```python
from build123d import *

# Parameters (mm, degrees)
F0_R            = 40
F2_DEPTH        = 10
F3_D            = 5.5
F3_CSINK_D      = 11.2
F3_CSINK_ANGLE  = 90
F3_COPIES_COUNT = 3
F4_R            = 4
F5_DEPTH        = 8
F5_COPIES_COUNT = 3
F6_SIZE         = 1


# Not quite as in the source:
# - a pattern or mirror of a feature is missing from the dataset's text; its kind, count and spacing are read off the source's solid
# - a feature names something its author has since deleted; it is built from what else it names


with BuildPart() as f2:
    # F0 (on Top) → F2 (new body)
    with BuildSketch(Plane.XY):
        Circle(F0_R)
    extrude(amount=-F2_DEPTH)

    # F3 (through all)
    with Locations(Plane.XY):
        with Locations((0, 18)):
            f3 = CounterSinkHole(F3_D / 2, F3_CSINK_D / 2, counter_sink_angle=F3_CSINK_ANGLE)

    # F3_copies: F3 ×3 about axis
    f3_copies_axis = Axis((0, 0, 0), (0, 0, 1))
    for i in range(1, F3_COPIES_COUNT):
        add(f3.rotate(f3_copies_axis, i * 360 / F3_COPIES_COUNT), mode=Mode.SUBTRACT)

    # F4 (on face) → F5 (cut)
    with BuildSketch(Plane.XY):
        with Locations((0, -10)):
            Circle(F4_R)
    f5 = extrude(amount=-F5_DEPTH, mode=Mode.SUBTRACT)

    # F5_copies: F5 ×3 about axis
    f5_copies_axis = Axis((0, 0, 0), (0, 0, 1))
    for i in range(1, F5_COPIES_COUNT):
        add(f5.rotate(f5_copies_axis, i * 360 / F5_COPIES_COUNT), mode=Mode.SUBTRACT)

    # F6
    f6_edges = [f2.edges().sort_by_distance(p)[0] for p in [
        (-40, 0, -10),
        (-40, 0, 0),
        (-4, -10, 0),
        (-6.660254, 8.464102, 0),
        (10.660254, 1.535898, 0),
    ]]
    chamfer(f6_edges, length=F6_SIZE)


solid = f2.part
```
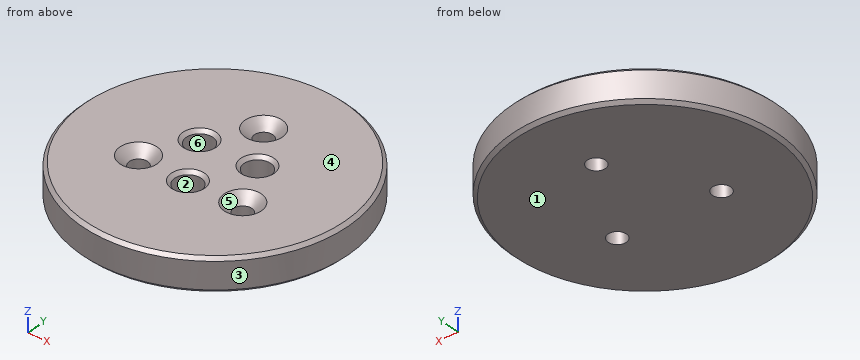
The model under review builds one solid part; all positions refer to its coordinate system, in mm. Face numbers are marked on the shaded views. A direction names the side the tool comes from. Give positions to 0.01 mm unless a question says otherwise; leave off trailing zeros. Write each loop counter-clockwise with the first axis right and the second up, starting at its lowest first coordinate (ties: lowest second). Pieces come first, ordered by that corner, then holes.
(1) Consider section A-A, the plane x = 0. Give the boundary of the cut face in (y, z).
(2) The part is to be moulded in two halves that separate along X. For the marked faces 3, 4, 5 and 6, say which applies: released by +X, released by -X, zero draft, split by the parting line, or undercut.
(3) Consider section B-B, the plane z = -4.75. Give the boundary of the cut face in (x, y), and give its area (3 significant figures).
(4) To check wall thickness, follow L1, parallel to Y at x = 0, z = -4.25; L2, parallel to Y at x = 3.5, z = -1.75; L3, parallel to X at y = -6.5, z = -6.5. State the ranges of each line that lie inside material, in increasing order.
(5) Tool access review of the marked faces 1 and 2: name each direction out of +Z, -Z, +X, -X, +Y, -Y from which nothing blocks a thin tool from reaching the whole face with its end or side.
(6) Consider section C-C, the plane y = -9. Give the number of separate pieces and of enclosed holes in the cut face, and give its area (3 significant figures).
(7) For P1, Ø5, axis at x = 0, y = -10, coming from the +Z side; P2, Ø2, axis at y = -2, z = -3.5, coming from the +X side; P3, Ø5, axis at y = 17.5, z = -8, coming from the -X side, all flat-tipped, find the tip position at first contact; note any pin that passes through.
Returned:
1. outline: (-40, -9) - (-39, -10) - (15.25, -10) - (15.25, -2.85) - (12.4, 0) - (-5, 0) - (-6, -1) - (-6, -8) - (-14, -8) - (-14, -1) - (-15, 0) - (-39, 0) - (-40, -1) - close; (20.75, -10) - (39, -10) - (40, -9) - (40, -1) - (39, 0) - (23.6, 0) - (20.75, -2.85) - close
2. face 3: split by the parting line
2. face 4: zero draft
2. face 5: undercut
2. face 6: undercut
3. outline: circle Ø80 at (0, 0); hole circle Ø5.5 at (-15.59, -9); hole circle Ø8 at (-8.66, 5); hole circle Ø8 at (0, -10); hole circle Ø5.5 at (0, 18); hole circle Ø8 at (8.66, 5); hole circle Ø5.5 at (15.59, -9)
3. area: 4,800 mm2
4. L1: y = -40 to -14, -6 to 15.25, 20.75 to 40
4. L2: y = -39.85 to -11.94, -8.06 to 16.4, 19.6 to 39.85
4. L3: x = -39.47 to -16.73, -14.44 to -1.94, 1.94 to 14.44, 16.73 to 39.47
5. face 1: -Z, +X, -X, +Y, -Y
5. face 2: +Z
6. separate pieces: 3
6. enclosed holes: 0
6. area: 588 mm2
7. P1: stops at z = -8
7. P2: stops at x = 39.99
7. P3: stops at x = -37.08
